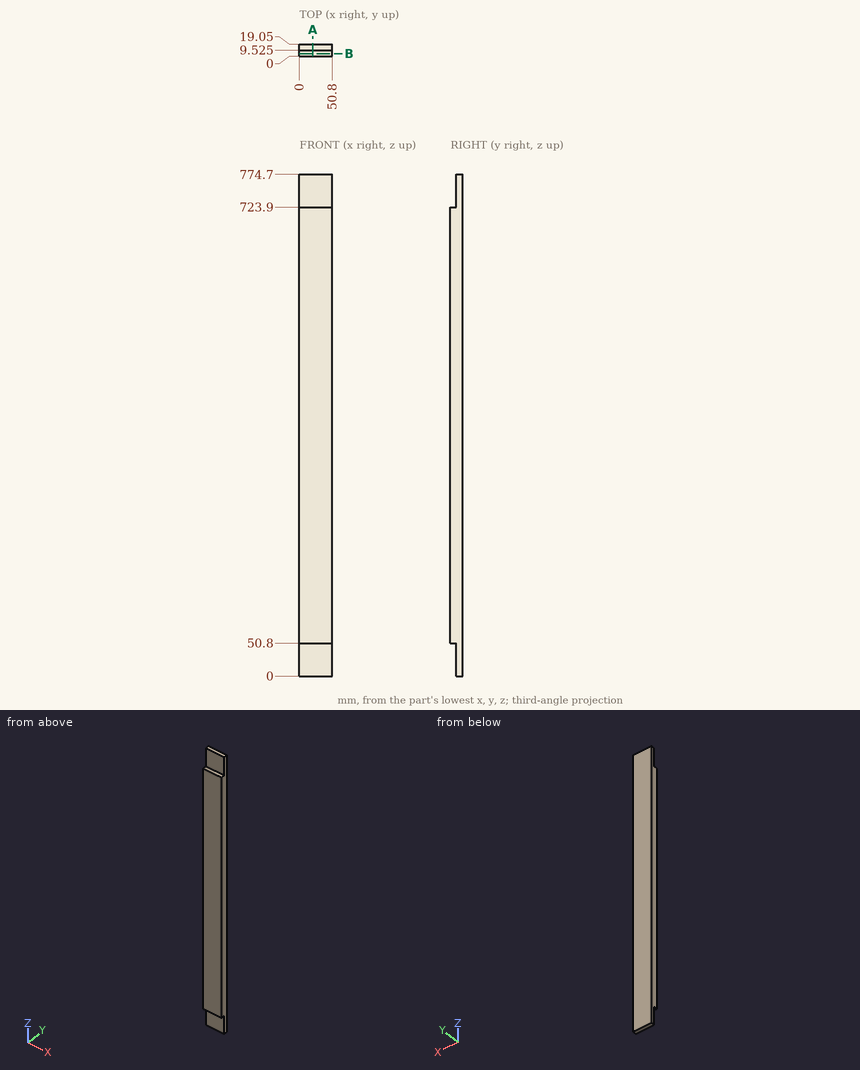
Source: three-view drawing plus pictorial views. Frame: mm from the lowest corner of the part. Round coordinates to 2 decimals unless told otherwise and drop trailing zeros. Loops run counter-clockwise (first coordinate to the right, second up) from the corner with the lowest first, then second, coordinate; pieces in that order, holes last. Notation, with made-up numbers: (80, -26) - (120, -26) arc R25 ccw to (120, -10) - close; hole circle Ø10 at (-20, 67.25). An arc over 180 degrees is marked (long way). Write item = value, one per line. Start each with the question number.
Item 1: Section query A-A on x = 21. Output: boundary loops of the cut face in (y, z) (3 decimals).
Item 2: Section query B-B on y = 4.25. Output: boundary loops of the cut face in (x, z), plus the area to 3 significant figures.
Item 3: First-contact query: pin 1 Ø8 at (x, y) = (36, 13.5) entering from -Z; pin 2 Ø1.5 at (x, y) = (30, 6) entering from -Z. Flat tips, straight axial feed; report the tip coordinate or a pass-through.
Item 4: Material intervals for line 1 (Z direction, x = 10, y = 7); line 2 (Y direction, x = 40, z = 725.5) (3 decimals), sorted ascending.
Results list:
q1.outline = (0, 50.8) - (9.525, 50.8) - (9.525, 0) - (19.05, 0) - (19.05, 774.7) - (9.525, 774.7) - (9.525, 723.9) - (0, 723.9) - close
q2.outline = (0, 50.8) - (50.8, 50.8) - (50.8, 723.9) - (0, 723.9) - close
q2.area = 34,200 mm²
q3.pin_1 = 0
q3.pin_2 = 50.8
q4.line_1 = 50.8 to 723.9
q4.line_2 = 9.525 to 19.05
